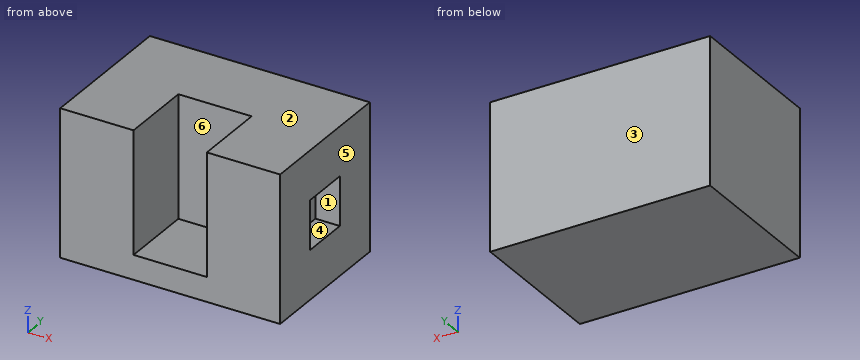
```python
from build123d import *

# Parameters (mm, degrees)
F0_W     = 228.6
F0_H     = 152.4
F1_DEPTH = 76.2
F2_W     = 50.8
F2_H     = 50.8
F3_DEPTH = 25.4
F4_W     = 76.2
F4_H     = 127
F5_DEPTH = 76.2


with BuildPart() as f1:
    # F0 (on Top) → F1 (new body, symmetric)
    with BuildSketch(Plane.XY):
        Rectangle(F0_W, F0_H)
    extrude(amount=F1_DEPTH, both=True)

    # F2 (on face) → F3 (cut)
    with BuildSketch(Plane.YZ.offset(114.3)):
        Rectangle(F2_W, F2_H)
    extrude(amount=-F3_DEPTH, mode=Mode.SUBTRACT)

    # F4 (on face) → F5 (cut)
    with BuildSketch(Plane.XZ.offset(76.2)):
        with Locations((0, 12.7)):
            Rectangle(F4_W, F4_H)
    extrude(amount=-F5_DEPTH, mode=Mode.SUBTRACT)


solid = f1.part
```
Geometry check sheet. Reference: the model listing, model coordinates, mm. Face numbers are marked on the shaded views. A direction names the side the tool comes from. Coordinates: 2 decimals unless noted, no trailing zeros. Order: outer loops, then holes, each group sorted by start corner. A loop starts at its lowest first (then second) coordinate and runs counter-clockwise, first axis right, second up. Notation, with made-up numbers: M 74.25,30.25 L 109.25,30.25 A18 ccw 109.25,64.25 Z; hole C 80.5,77.25 d10. An arc over 180 degrees is marked long. One line per question, with ' | ' between items. Start each with the question number.
Item 1: Cross-section at B-B on z = 7. Enter the section's corners in (x, y), then the cut area to 3 significant figures.
Item 2: Cross-section at D-D on y = -3. Enter the section's corners in (x, z).
Item 3: Cross-section at C-C on z = -34.5. Enter the section's corners in (x, y).
Item 4: Material ranges on L1, parallel to X at y = -52, z = -7.5; L2, parallel to Y at x = -21, z = 16; L3, parallel to X at y = 6.5, z = -22, recorded low to high. Write a range as [from, to].
Item 5: Draft check along Z on the marked faces 1, 2 and 3. Enter one of: pulls with the +Z half, pulls with the -Z half, needs draft (parallel to the pull), parting line crosses it, or undercut.
Item 6: Gauge pin test, flat end, axial feed: pin 1 (1.5 mm diameter, centred on x = 21, y = -32, fed in from +Z). Record the tip position at first contact, or that the pin passes through.
Item 7: Set-up check for the marked faces 4, 5 and 6: record each of +Z, -Z, +X, -X, +Y, -Y from which the full face is reachable in a straight line by a thin tool's end or side.
Item 8: Cross-section at A-A on y = -31.5. Enter the section's corners in (x, z), then the cut area to 3 significant figures.
Findings:
1) outline: M -114.3,-76.2 L -38.1,-76.2 L -38.1,0 L 38.1,0 L 38.1,-76.2 L 114.3,-76.2 L 114.3,-25.4 L 88.9,-25.4 L 88.9,25.4 L 114.3,25.4 L 114.3,76.2 L -114.3,76.2 Z | area: 27,700 mm²
2) outline: M -114.3,-76.2 L 114.3,-76.2 L 114.3,-25.4 L 88.9,-25.4 L 88.9,25.4 L 114.3,25.4 L 114.3,76.2 L 38.1,76.2 L 38.1,-50.8 L -38.1,-50.8 L -38.1,76.2 L -114.3,76.2 Z
3) outline: M -114.3,-76.2 L -38.1,-76.2 L -38.1,0 L 38.1,0 L 38.1,-76.2 L 114.3,-76.2 L 114.3,76.2 L -114.3,76.2 Z
4) L1: x = [-114.3, -38.1], [38.1, 114.3] | L2: y = [0, 76.2] | L3: x = [-114.3, 88.9]
5) face 1: undercut | face 2: pulls with the +Z half | face 3: needs draft
6) pin 1: stops at z = -50.8
7) face 4: +X | face 5: +Z, -Z, +X, +Y, -Y | face 6: +Z, -Y
8) outline: M -114.3,-76.2 L 114.3,-76.2 L 114.3,76.2 L 38.1,76.2 L 38.1,-50.8 L -38.1,-50.8 L -38.1,76.2 L -114.3,76.2 Z | area: 25,200 mm²
